Geometry check sheet. Reference: the model listing, model coordinates, mm. Face numbers are marked on the shaded views. A direction names the side the tool comes from. Round coordinates to 2 decimals unless told otherwise and drop trailing zeros. Loops run counter-clockwise (first coordinate to the right, second up) from the corner with the lowest first, then second, coordinate; pieces in that order, holes last. Notation, with made-up numbers: (3, 38.25) -> (58, 38.25) arc R13 ccw to (58, 46.25) -> close; hole circle Ø1 at (80, 77). An arc over 180 degrees is marked (long way). Use one line per item in the form item = value.
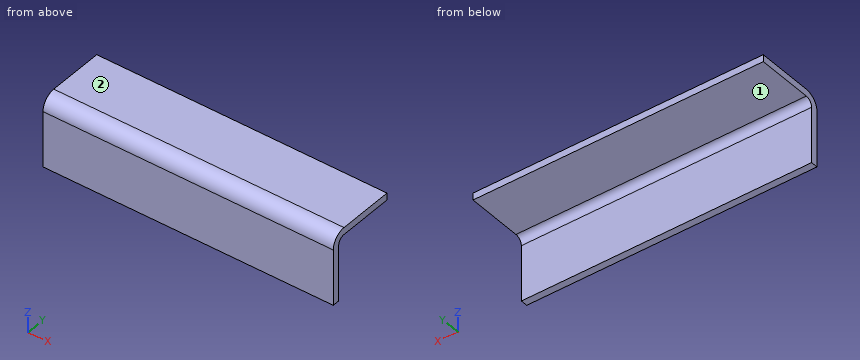
from build123d import *

# Parameters (mm, degrees)
SKETCH1_W                    = 250
SKETCH1_H                    = 60
BOSS_EXTRUDE1_DEPTH          = 4
CONVERT_SOLID1_START         = -125
CONVERT_SOLID1_OUTLINE_W     = 2
CONVERT_SOLID1_OUTLINE_H     = 60
CONVERT_SOLID1_DEPTH         = 250
EDGE_FLANGE1_STRIP_W         = 36
EDGE_FLANGE1_STRIP_H         = 6
EDGE_FLANGE1_STRIP_CUT_DEPTH = 250
EDGE_FLANGE1_DEPTH           = 250


# Read off the part's stored shape, not the designer's step: Convert-Solid1
# Sheet-metal steps are written as plain solids
with BuildPart() as part:
    # Sketch1 → Boss-Extrude1 (new body)
    with BuildSketch(Plane(origin=(0, 0, 0), x_dir=(1, 0, 0), z_dir=(0, 1, 0))):
        Rectangle(SKETCH1_W, SKETCH1_H)
    extrude(amount=BOSS_EXTRUDE1_DEPTH)

    # Convert-Solid1 outline → Convert-Solid1 (add)
    with BuildSketch(Plane.YZ.offset(CONVERT_SOLID1_START)):
        with Locations((-1, 0)):
            Rectangle(CONVERT_SOLID1_OUTLINE_W, CONVERT_SOLID1_OUTLINE_H)
    extrude(amount=CONVERT_SOLID1_DEPTH)

    # Edge-Flange1 strip (across the edge) → Edge-Flange1 strip cut (cut)
    with BuildSketch(Plane(origin=(-125, 4, 30), x_dir=(0, 0, -1), z_dir=(1, 0, 0))):
        with Locations((-6, -3)):
            Rectangle(EDGE_FLANGE1_STRIP_W, EDGE_FLANGE1_STRIP_H)
    extrude(amount=EDGE_FLANGE1_STRIP_CUT_DEPTH, mode=Mode.SUBTRACT)

    # Edge-Flange1 section (across the edge) → Edge-Flange1 (add)
    with BuildSketch(Plane(origin=(-125, 4, 30), x_dir=(0, 0, -1), z_dir=(1, 0, 0))):
        with BuildLine():
            Line((0, 6), (0, 54))
            Line((0, 54), (6, 54))
            Line((6, 54), (6, 6))
            ThreePointArc((6, 6), (7.757359313, 1.757359313), (12, 0))
            Line((12, 0), (12, -6))
            ThreePointArc((12, -6), (3.514718626, -2.485281374), (0, 6))
        make_face()
    extrude(amount=EDGE_FLANGE1_DEPTH)


solid = part.part
1. Section check C-C (y = 43). Record the boundary of the cut face in (x, z).
Return value:
outline = (-125, 24) -> (125, 24) -> (125, 30) -> (-125, 30) -> close
2. Section check B-B (z = -22.5). Record the boundary of the cut face in (x, y).
Return value:
outline = (-125, -2) -> (125, -2) -> (125, 4) -> (-125, 4) -> close
3. Tool access check on the marked faces 1 and 2. Record the directions out of +Z, -Z, +X, -X, +Y, -Y that give a thin tool (end or side, any length) a straight path to the whole face; none if there is none.
Return value:
face_1 = -Z, +X, -X, +Y
face_2 = +Z, +X, -X, +Y, -Y
4. Gauge pin test, flat ends, axial feed: pin 1 (2 mm diameter, centred on x = -39.5, y = 24.5, fed in from -Z); pin 2 (1.5 mm diameter, centred on x = -20.5, z = 23, fed in from -Y). Record the tip position at first contact, or that the pin passes through.
Return value:
pin_1 = 24
pin_2 = -1.22
5. Material ranges on line 1 along Z through (x, y) = (-44.5, 49.5); line 2 along Y through (x, z) = (-2, 16.5); line 3 along Z through (x, y) = (-22, 8.5), recorded low to high.
Return value:
line_1 = 24 to 30
line_2 = -2 to 4
line_3 = 23.81 to 29.91
6. Section check A-A (x = 72). Record the boundary of the cut face in (y, z).
Return value:
outline = (-2, -30) -> (4, -30) -> (4, 18) arc R6 cw to (10, 24) -> (58, 24) -> (58, 30) -> (10, 30) arc R12 ccw to (-2, 18) -> close
